from build123d import *

# Parameters (mm, degrees)
F0_W     = 124.060318
F0_H     = 61.61835
F1_DEPTH = 25.4
F2_R     = 17.541001
F3_DEPTH = 25.4
F5_DEPTH = 61.61935


with BuildPart() as f1:
    # F0 (on Front) → F1 (new body)
    with BuildSketch(Plane.XZ):
        Rectangle(F0_W, F0_H)
    extrude(amount=F1_DEPTH)

    # F2 (on face) → F3 (join)
    with BuildSketch(Plane(origin=(0, 0, 0), x_dir=(-1, 0, 0), z_dir=(0, 1, 0))):
        with Locations((-17.289521, -2.959591)):
            Circle(F2_R)
    extrude(amount=F3_DEPTH)

    # F4 (on face) → F5 (cut, through all)
    with BuildSketch(Plane(origin=(0, 0, -30.809175), x_dir=(1, 0, 0), z_dir=(0, 0, -1))):
        Polygon((-0.25148, -25.4), (34.830522, -25.4), (-0.25148, 0), align=None)
    extrude(amount=-F5_DEPTH, mode=Mode.SUBTRACT)


solid = f1.part
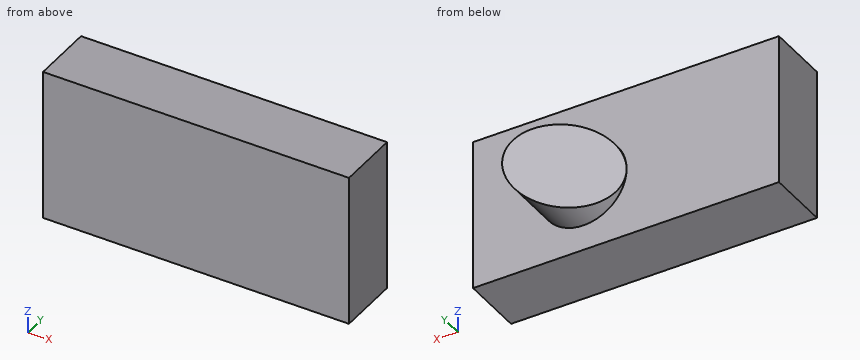
Model file for the job. Use its own axes, mm. Round coordinates to 2 decimals unless told otherwise and drop trailing zeros. Loops run counter-clockwise (first coordinate to the right, second up) from the corner with the lowest first, then second, coordinate; pieces in that order, holes last. Notation, with made-up numbers: M 57,-15.75 L 80,-15.75 A33 cw 80,21.25 Z; hole C 69,10.25 d10. An arc over 180 degrees is marked long. One line per question, with ' | ' between items.
1) Band-saw the part on B-B (x = 23). Give the cut face in (y, z), then the cut area to 3 significant figures.
Solved:
outline: M -25.4,-30.81 L 0,-30.81 L 0,-19.55 L 16.83,-19.55 L 16.83,13.63 L 0,13.63 L 0,30.81 L -25.4,30.81 Z | area: 2,120 mm²
2) Flat gauge pins, fed straight in: pin 1 (12 mm diameter, centred on y = 16.5, z = -15, fed in from -X); pin 2 (5 mm diameter, centred on y = 15, z = -3.5, fed in from -X); pin 3 (1.5 mm diameter, centred on x = 4, y = 6, fed in from -Z); pin 4 (3 mm diameter, centred on x = 6.5, z = -12.5, fed in from +Y). Where does each tip first touch, or does it go through?
Solved:
pin 1: stops at x = 14.25 | pin 2: stops at x = 17.01 | pin 3: passes through | pin 4: stops at y = 5.97
3) Band-saw the part on D-D (x = 39). Give the cut face in (y, z).
Solved:
outline: M -25.4,-30.81 L 0,-30.81 L 0,30.81 L -25.4,30.81 Z
4) Band-saw the part on C-C (y = 10.5). Give the cut face in (x, z).
Solved:
outline: M 14.25,-20.24 A17.54 ccw long 14.25,14.32 Z
5) Drill centre lines: line 1 along Y through (x, z) = (-17.5, -11); line 2 along X through (y, z) = (20, 0); line 3 along Z through (x, y) = (3, 1). Where is each one in solid material? Low to high.
Solved:
line 1: y = -25.4 to 0 | line 2: x = 27.37 to 34.58 | line 3: z = -13.13 to 7.21
6) Band-saw the part on A-A (z = -19). Give the cut face in (x, y), then the cut area to 3 significant figures.
Solved:
outline: M -62.03,-25.4 L 62.03,-25.4 L 62.03,0 L 24.39,0 L 24.39,17.84 L 10.19,7.56 L 10.19,0 L -62.03,0 Z | area: 3,330 mm²
